Answer from the drawing. Dimensions are ordinates in mm from the lowest x, y and z of the part. Round coordinates to 2 decimals unless told otherwise and drop trailing zeros. Order: outer loops, then holes, each group sorted by start corner. A loop starts at its lowest first (then second) coordinate and runs counter-clockwise, first axis right, second up. Notation, with made-up numbers: (20, -35) - (47, -35) arc R21 ccw to (47, -29) - close; hole circle Ø9 at (35, 16). An arc over 180 degrees is marked (long way). One line per question, with ' | ' between items. Start each with the question number.
1) The part is cut by section B-B, the plane y = 5. Give the vertices of the cut face in (x, z) (1 decimal), plus the area to 3 significant figures.
2) Straight lines are drawn through the part: line 1 (Y direction, x = 4.5, z = 0.5) (1 decimal); line 2 (X direction, y = 1.75, z = 0.3); line 3 (Y direction, x = 4.75, z = 0.6) (1 decimal). For each, find the intervals that lie inside material, in ascending order. Write a range as from..to.
3) The part is cut by section A-A, the plane z = 0.55. Give the vertices of the cut face in (x, y) (1 decimal), plus the area to 3 significant figures.
4) The part is cut by section C-C, the plane x = 15.25. Give the vertices of the cut face in (y, z).
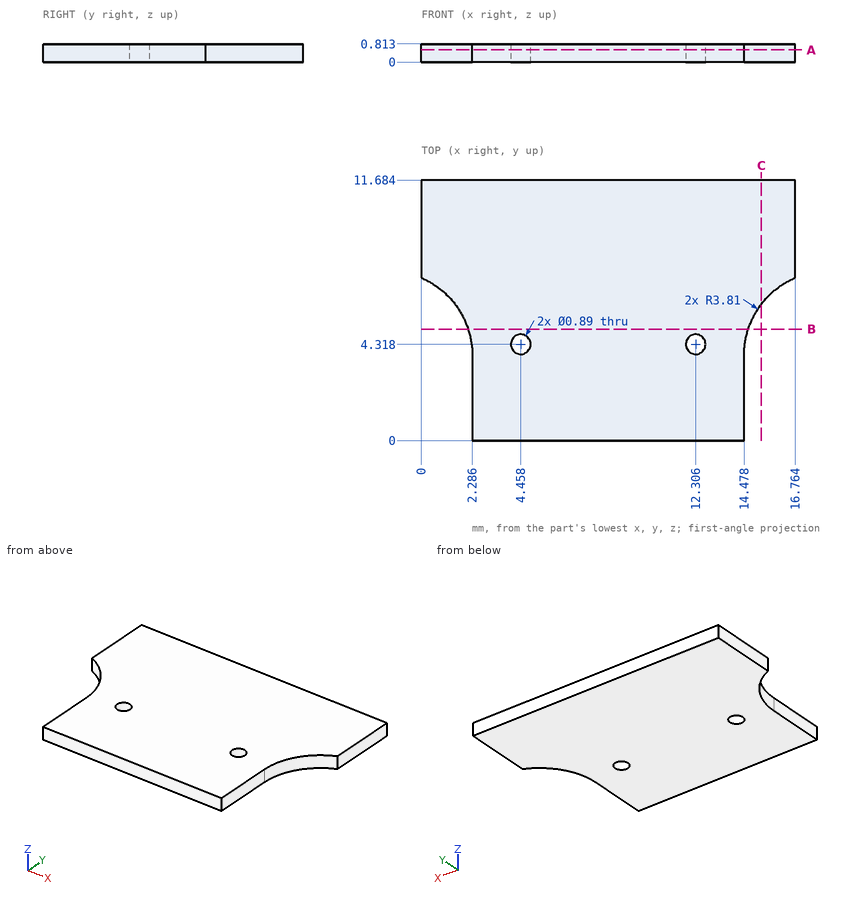
Values:
1) outline: (2.1, 0) - (14.7, 0) - (14.7, 0.8) - (2.1, 0.8) - close | area: 10.2 mm^2
2) line 1: y = 0..3.9, 4.8..11.7 | line 2: x = 2.29..14.48 | line 3: y = 0..4, 4.7..11.7
3) outline: (0, 7.3) arc R3.8 cw to (2.3, 3.8) - (2.3, 0) - (14.5, 0) - (14.5, 3.8) arc R3.8 cw to (16.8, 7.3) - (16.8, 11.7) - (0, 11.7) - close; hole circle Ø0.9 at (4.5, 4.3); hole circle Ø0.9 at (12.3, 4.3) | area: 166 mm^2
4) outline: (6.11, 0) - (11.68, 0) - (11.68, 0.81) - (6.11, 0.81) - close
